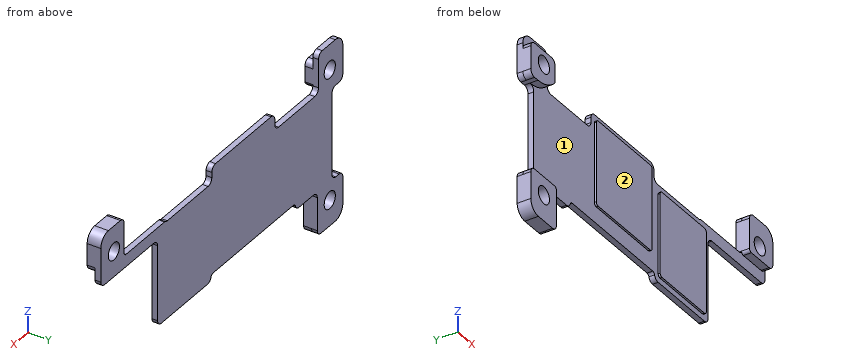
```python
from build123d import *

# Parameters (mm, degrees)
BOSS_EXTRUDE1_START = 1.4
SKETCH2_R           = 1.5
BOSS_EXTRUDE1_DEPTH = 1
SKETCH4_W           = 51.3
SKETCH4_H           = 7.828136
CUT_EXTRUDE1_DEPTH  = 37.239562
SKETCH5_W           = 15.253092
SKETCH5_H           = 23.040436
CUT_EXTRUDE2_DEPTH  = 37.239562
SKETCH6_W           = 22.069426
SKETCH6_H           = 6.8
SKETCH6_W_2         = 11.75
SKETCH6_H_2         = 7
CUT_EXTRUDE3_DEPTH  = 37.239562
SKETCH7_W           = 2.92226
SKETCH7_H           = 16.173552
SKETCH7_W_2         = 22.599024
SKETCH7_H_2         = 1.175102
CUT_EXTRUDE4_DEPTH  = 37.239562
FILLET8_R           = 1
FILLET10_R          = 0.5
SKETCH9_W           = 12.4
SKETCH9_H           = 15
SKETCH9_W_2         = 15
BOSS_EXTRUDE2_DEPTH = 0.35
FILLET3_R           = 0.5
BOSS_EXTRUDE3_START = -2.4
SKETCH10_R          = 1.5
BOSS_EXTRUDE3_DEPTH = 2.4
FILLET6_R           = 0.5
FILLET11_R          = 1
FILLET13_R          = 0.5


with BuildPart() as part:
    # Sketch2 → Boss-Extrude1 (new body)
    with BuildSketch(Plane(origin=(0, 0, 0), x_dir=(1, 0, 0), z_dir=(0, 1, 0)).offset(BOSS_EXTRUDE1_START)):
        with BuildLine():
            Line((-32.500062, 13.969619), (-32.500062, -13.969619))
            ThreePointArc((-32.500062, -13.969619), (-31.904903, -15.40646), (-30.468062, -16.001619))
            Line((-30.468062, -16.001619), (30.468062, -16.001619))
            ThreePointArc((30.468062, -16.001619), (31.904903, -15.40646), (32.500062, -13.969619))
            Line((32.500062, -13.969619), (32.500062, 13.969619))
            ThreePointArc((32.500062, 13.969619), (31.904903, 15.40646), (30.468062, 16.001619))
            Line((30.468062, 16.001619), (-30.468062, 16.001619))
            ThreePointArc((-30.468062, 16.001619), (-31.904903, 15.40646), (-32.500062, 13.969619))
        make_face()
        with Locations(Location((28.999942, 11.463655, 0), (0, 0, 270))):
            Circle(SKETCH2_R, mode=Mode.SUBTRACT)
        with Locations(Location((28.999942, -11.536299, 0), (0, 0, 270))):
            Circle(SKETCH2_R, mode=Mode.SUBTRACT)
        with Locations(Location((-29.000196, -11.536299, 0), (0, 0, 270))):
            Circle(SKETCH2_R, mode=Mode.SUBTRACT)
        with Locations(Location((-29.000196, 11.463655, 0), (0, 0, 270))):
            Circle(SKETCH2_R, mode=Mode.SUBTRACT)
    extrude(amount=BOSS_EXTRUDE1_DEPTH)

    # Sketch4 → Cut-Extrude1 (cut, through all)
    with BuildSketch(Plane(origin=(0, 2.4, 0), x_dir=(1, 0, 0), z_dir=(0, 1, 0))):
        with Locations((0.010922, 12.087551)):
            Rectangle(SKETCH4_W, SKETCH4_H)
    extrude(amount=-CUT_EXTRUDE1_DEPTH, mode=Mode.SUBTRACT)

    # Sketch5 → Cut-Extrude2 (cut, through all)
    with BuildSketch(Plane(origin=(0, 2.4, 0), x_dir=(1, 0, 0), z_dir=(0, 1, 0))):
        with Locations((24.873516, 4.481401)):
            Rectangle(SKETCH5_W, SKETCH5_H)
    extrude(amount=-CUT_EXTRUDE2_DEPTH, mode=Mode.SUBTRACT)

    # Sketch6 → Cut-Extrude3 (cut, through all)
    with BuildSketch(Plane(origin=(0, 2.4, 0), x_dir=(1, 0, 0), z_dir=(0, 1, 0))):
        with Locations((15.204059, -12.601619)):
            Rectangle(SKETCH6_W, SKETCH6_H)
        with Locations((-20.100036, -12.501619)):
            Rectangle(SKETCH6_W_2, SKETCH6_H_2)
    extrude(amount=-CUT_EXTRUDE3_DEPTH, mode=Mode.SUBTRACT)

    # Sketch7 → Cut-Extrude4 (cut, through all)
    with BuildSketch(Plane(origin=(0, 2.4, 0), x_dir=(1, 0, 0), z_dir=(0, 1, 0))):
        Polygon((2.69737, -11.925317), (2.69737, -9.001619), (15.24697, -9.001619), (15.24697, -16.001619), (-14.225036, -16.001619), (-14.225036, -11.925317), align=None)
        with Locations((-31.038932, 0.152527)):
            Rectangle(SKETCH7_W, SKETCH7_H)
        with Locations((-8.452542, 7.585932)):
            Rectangle(SKETCH7_W_2, SKETCH7_H_2)
    extrude(amount=-CUT_EXTRUDE4_DEPTH, mode=Mode.SUBTRACT)

    # Fillet8
    # the kernel refuses this fillet: 1 mm, written as the material it adds along each edge
    with BuildSketch(Plane(origin=(15.24697, 2.4, 9.001619), x_dir=(0, 0, 1), z_dir=(0, -1, 0))) as fillet8_piece_1:
        with BuildLine():
            CenterArc((1, 0.6), FILLET8_R, 180, 36.869898)
            Line((0, 0.6), (0, 0))
            Line((0, 0), (0.2, 0))
        make_face()
    extrude(amount=1)
    with BuildSketch(Plane(origin=(-29.577802, 2.4, 7.934249), x_dir=(-1, 0, 0), z_dir=(0, -1, 0)), Plane(origin=(-25.975036, 2.4, 9.001619), x_dir=(1, 0, 0), z_dir=(0, -1, 0)), Plane(origin=(-14.225036, 2.4, 9.001619), x_dir=(0, 0, 1), z_dir=(0, -1, 0)), Plane(origin=(2.69737, 2.4, 9.001619), x_dir=(1, 0, 0), z_dir=(0, -1, 0)), Plane(origin=(17.24697, 2.4, 7.038817), x_dir=(0, 0, -1), z_dir=(0, -1, 0)), Plane(origin=(-25.639078, 2.4, -8.173483), x_dir=(0, 0, -1), z_dir=(0, -1, 0)), Plane(origin=(-29.577802, 2.4, -8.239303), x_dir=(0, 0, 1), z_dir=(0, -1, 0))) as fillet8_piece_2:
        with BuildLine():
            CenterArc((FILLET8_R, FILLET8_R), FILLET8_R, 180, 90)
            Line((0, FILLET8_R), (0, 0))
            Line((0, 0), (FILLET8_R, 0))
        make_face()
    extrude(amount=1)
    # the kernel refuses this fillet: 1 mm, written as the material it takes off along each edge
    with BuildSketch(Plane(origin=(-32.500062, 4.9, 7.934249), x_dir=(0, 0, 1), z_dir=(0, -1, 0)), Plane(origin=(-25.975036, 4.9, 16.001619), x_dir=(0, 0, -1), z_dir=(0, -1, 0)), Plane(origin=(-14.225036, 4.9, 11.925317), x_dir=(1, 0, 0), z_dir=(0, -1, 0)), Plane(origin=(2.69737, 4.9, 11.925317), x_dir=(0, 0, -1), z_dir=(0, -1, 0)), Plane(origin=(26.238772, 4.9, 16.001619), x_dir=(1, 0, 0), z_dir=(0, -1, 0)), Plane(origin=(2.84697, 4.9, -8.173483), x_dir=(0, 0, 1), z_dir=(0, -1, 0)), Plane(origin=(-19.752054, 4.9, -8.173483), x_dir=(-1, 0, 0), z_dir=(0, -1, 0)), Plane(origin=(-25.639078, 4.9, -16.001619), x_dir=(-1, 0, 0), z_dir=(0, -1, 0)), Plane(origin=(-32.500062, 4.9, -8.239303), x_dir=(1, 0, 0), z_dir=(0, -1, 0)), Plane(origin=(32.500062, 4.9, 7.038817), x_dir=(-1, 0, 0), z_dir=(0, -1, 0))) as fillet8_2_piece_1:
        with BuildLine():
            CenterArc((FILLET8_R, -FILLET8_R), FILLET8_R, 90, 90)
            Line((0, -FILLET8_R), (0, 0))
            Line((0, 0), (FILLET8_R, 0))
        make_face()
    extrude(amount=6, mode=Mode.SUBTRACT)
    with BuildSketch(Plane(origin=(17.24697, -1.1, -8.173483), x_dir=(-1, 0, 0), z_dir=(0, 1, 0))) as fillet8_2_piece_2:
        with BuildLine():
            CenterArc((FILLET8_R, FILLET8_R), FILLET8_R, 180, 90)
            Line((0, FILLET8_R), (0, 0))
            Line((0, 0), (FILLET8_R, 0))
        make_face()
    extrude(amount=6, mode=Mode.SUBTRACT)

    # Fillet10
    fillet10_edges = [part.edges().sort_by_distance(p)[0] for p in [
        (26.238772, 1.9, 9.201619),
    ]]
    fillet(fillet10_edges, radius=FILLET10_R)

    # Sketch9 → Boss-Extrude2 (add)
    with BuildSketch(Plane.XZ.offset(-1.4)):
        with Locations((10.04697, 0.326517)):
            Rectangle(SKETCH9_W, SKETCH9_H)
        with Locations((-5.80263, 3.425317)):
            Rectangle(SKETCH9_W_2, SKETCH9_H)
    extrude(amount=BOSS_EXTRUDE2_DEPTH)

    # Fillet3
    fillet3_edges = [part.edges().sort_by_distance(p)[0] for p in [
        (16.24697, 1.225, 7.826517),
        (3.84697, 1.225, 7.826517),
        (3.84697, 1.225, -7.173483),
        (16.24697, 1.225, -7.173483),
        (1.69737, 1.225, 10.925317),
        (-13.30263, 1.225, 10.925317),
        (-13.30263, 1.225, -4.074683),
        (1.69737, 1.225, -4.074683),
    ]]
    fillet(fillet3_edges, radius=FILLET3_R)

    # Sketch10 → Boss-Extrude3 (add)
    # profile 1 of 3: a face of its own
    with BuildSketch(Plane(origin=(0, 2.4, 0), x_dir=(1, 0, 0), z_dir=(0, 1, 0)).offset(BOSS_EXTRUDE3_START)):
        with BuildLine():
            Line((-30.577802, 8.239303), (-25.639078, 8.239303))
            Line((-25.639078, 8.239303), (-25.639078, 9.173483))
            Line((-25.639078, 9.173483), (-25.639078, 15.001619))
            ThreePointArc((-25.639078, 15.001619), (-25.931971, 15.708726), (-26.639078, 16.001619))
            Line((-26.639078, 16.001619), (-30.468062, 16.001619))
            ThreePointArc((-30.468062, 16.001619), (-31.904903, 15.40646), (-32.500062, 13.969619))
            Line((-32.500062, 13.969619), (-32.500062, 9.239303))
            ThreePointArc((-32.500062, 9.239303), (-32.207169, 8.532196), (-31.500062, 8.239303))
            Line((-31.500062, 8.239303), (-30.577802, 8.239303))
        make_face()
        with Locations(Location((-29.000196, 11.463655, 0), (0, 0, 270))):
            Circle(SKETCH10_R, mode=Mode.SUBTRACT)
    # profile 2 of 3: a face of its own
    with BuildSketch(Plane(origin=(0, 2.4, 0), x_dir=(1, 0, 0), z_dir=(0, 1, 0)).offset(BOSS_EXTRUDE3_START)):
        with BuildLine():
            Line((-25.975036, -10.001619), (-25.975036, -13.958671))
            Line((-25.975036, -13.958671), (-32.500062, -13.958671))
            Line((-32.500062, -13.958671), (-32.500062, -8.934249))
            ThreePointArc((-32.500062, -8.934249), (-32.207169, -8.227142), (-31.500062, -7.934249))
            Line((-31.500062, -7.934249), (-30.577802, -7.934249))
            ThreePointArc((-30.577802, -7.934249), (-28.054933, -8.47482), (-25.975036, -10.001619))
        make_face()
        with Locations(Location((-29.000196, -11.536299, 0), (0, 0, 270))):
            Circle(SKETCH10_R, mode=Mode.SUBTRACT)
    # profile 3 of 3: a face of its own
    with BuildSketch(Plane(origin=(0, 2.4, 0), x_dir=(1, 0, 0), z_dir=(0, 1, 0)).offset(BOSS_EXTRUDE3_START)):
        with BuildLine():
            Line((26.238772, -9.701619), (26.238772, -9.185593))
            Line((26.238772, -9.185593), (32.500062, -9.185593))
            Line((32.500062, -9.185593), (32.500062, -13.969619))
            ThreePointArc((32.500062, -13.969619), (31.904903, -15.40646), (30.468062, -16.001619))
            Line((30.468062, -16.001619), (27.238772, -16.001619))
            ThreePointArc((27.238772, -16.001619), (26.531665, -15.708726), (26.238772, -15.001619))
            Line((26.238772, -15.001619), (26.238772, -9.701619))
        make_face()
        with Locations(Location((28.999942, -11.536299, 0), (0, 0, 270))):
            Circle(SKETCH10_R, mode=Mode.SUBTRACT)
    extrude(amount=BOSS_EXTRUDE3_DEPTH)

    # Fillet6
    fillet6_edges = [part.edges().sort_by_distance(p)[0] for p in [
        (15.24697, 1.9, 9.201619),
        (2.84697, 1.9, -6.998381),
        (-19.752054, 1.9, -6.998381),
        (-25.639078, 0.7, -8.239303),
    ]]
    fillet(fillet6_edges, radius=FILLET6_R)

    # Fillet11
    fillet11_edges = [part.edges().sort_by_distance(p)[0] for p in [
        (-25.975036, 0.7, 13.958671),
        (-32.500062, 0.7, 13.958671),
        (32.500062, 0.7, 9.185593),
    ]]
    fillet(fillet11_edges, radius=FILLET11_R)

    # Fillet13
    fillet13_edges = [part.edges().sort_by_distance(p)[0] for p in [
        (-25.975036, 0.7, 10.001619),
        (26.238772, 0.7, 9.185593),
    ]]
    fillet(fillet13_edges, radius=FILLET13_R)


solid = part.part
```
Can you work these out from the model? Positions are in its coordinate system, mm. Face numbers are marked on the shaded views. Give positions to 0.01 mm unless a question says otherwise; leave off trailing zeros. Loops run counter-clockwise (first coordinate to the right, second up) from the corner with the lowest first, then second, coordinate; pieces in that order, holes last. Notation, with made-up numbers: M 32.5,5 L 67.5,5 A22 cw 67.5,24 Z; hole C 21,23 d3. An arc over 180 degrees is marked long. Use one line per item in the form item = value. Start each with the question number.
(1) Thinking about a two-plate mould opening in Z: for the marked faces 1 and 2, which applies, released by +Z, released by -Z, zero draft, split by the parting line, or undercut?
(2) I'm going to push flat-ended pins straight in: P1, Ø2.5, axis at x = 29, z = 11.54, coming from the -Y side; P2, Ø4.5, axis at x = -3.5, z = 4.5, coming from the -Y side; P3, Ø0.7, axis at x = 28.5, y = 1, coming from the -Z side; P4, Ø1.2, axis at x = -29, y = 1, coming from the +Z side. Where does each tip first touch, or does it pass through?
(3) I want a section at D-D, the plane x = -23. Write out the boundary of the cut face in (y, z), and give its area (3 significant figures).
(4) I want a section at A-A, the plane y = 0.55. Write out the boundary of the cut face in (x, z).
(5) I want a section at C-C, the plane z = 1. Write out the boundary of the cut face in (x, y).
(6) Please list where these lines run through material, in increasing order: line 1 (X direction, y = 1.25, z = 7); line 2 (Z direction, x = 15.5, y = 1.75); line 3 (X direction, y = 2.2, z = -0.5).
(7) I want a section at B-B, the plane x = 11.5. Write out the boundary of the cut face in (y, z).
Worked out:
q1.face_1 = undercut
q1.face_2 = zero draft
q2.P1 = through
q2.P2 = 1.05
q2.P3 = 9.19
q2.P4 = 16
q3.outline = M 1.4,-8.17 L 2.4,-8.17 L 2.4,9 L 1.4,9 Z
q3.area = 17.2 mm²
q4.outline = M -32.5,-13.97 A2.03 ccw -30.47,-16 L -26.64,-16 A1 ccw -25.64,-15 L -25.64,-8.74 A0.5 ccw -26.14,-8.24 L -31.5,-8.24 A1 ccw -32.5,-9.24 Z; M -32.5,8.93 A1 ccw -31.5,7.93 L -30.58,7.93 A6.16 ccw -26.11,9.85 A0.5 ccw -25.98,10.2 L -25.98,12.96 A1 ccw -26.98,13.96 L -31.5,13.96 A1 ccw -32.5,12.96 Z; M 26.24,9.69 A0.5 ccw 26.74,9.19 L 31.5,9.19 A1 ccw 32.5,10.19 L 32.5,13.97 A2.03 ccw 30.47,16 L 27.24,16 A1 ccw 26.24,15 Z; hole C -29,-11.46 d3; hole C -29,11.54 d3; hole C 29,11.54 d3
q5.outline = M -29.58,1.4 L -13.3,1.4 L -13.3,1.05 L 1.7,1.05 L 1.7,1.4 L 3.85,1.4 L 3.85,1.05 L 16.25,1.05 L 16.25,1.4 L 17.25,1.4 L 17.25,2.4 L -29.58,2.4 Z
q6.line_1 = -13.3 to 1.7, 3.85 to 16.25
q6.line_2 = -8.17 to 9.2
q6.line_3 = -29.58 to 17.25
q7.outline = M 1.05,-7.17 L 1.4,-7.17 L 1.4,-8.17 L 2.4,-8.17 L 2.4,9 L 1.4,9 L 1.4,7.83 L 1.05,7.83 Z
